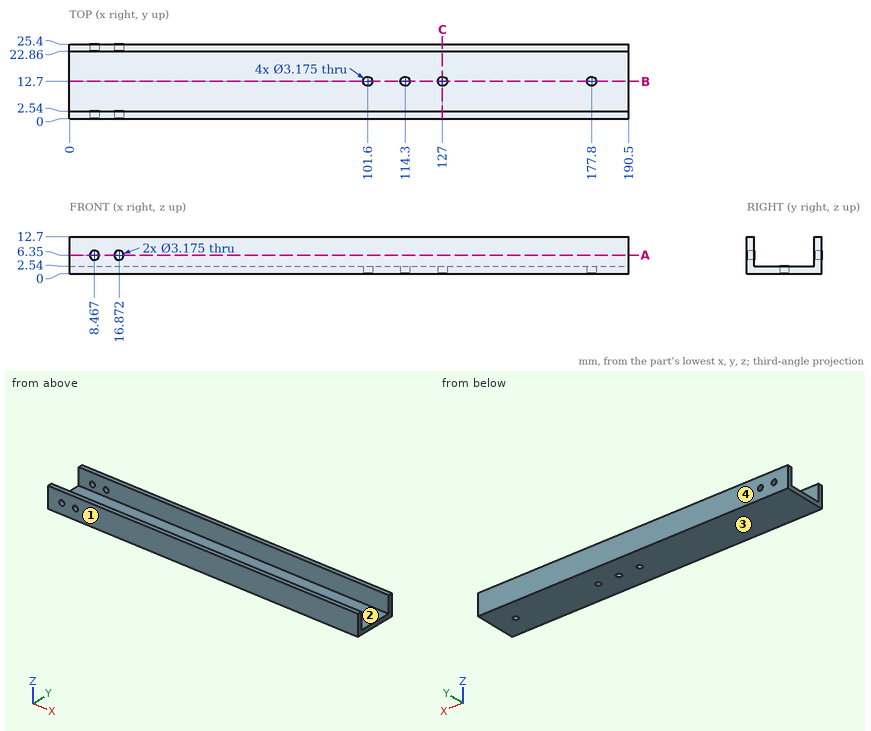
Geometry: see drawing. Coordinates: mm, zero at the bounding-box minimum. Give positions to 0.01 mm unless a question says otherwise; leave off trailing zeros. Order: outer loops, then holes, each group sorted by start corner. A loop starts at its lowest first (then second) coordinate and runs counter-clockwise, first axis right, second up. Notation, with made-up numbers: (50.5, 84) -> (54.5, 84) arc R23 ccw to (54.5, 122) -> close; hole circle Ø5 at (-4.5, -37.5). An arc over 180 degrees is marked (long way). Write each question's results on one line, items separated by ' | '. Start each with the question number.
1) Section A-A (z = 6.35). Return loops of the section in (x, y) (1 decimal).
2) Draft query along Y for the marked faces 1, 2, 3 and 4. Return one class per face: pulls with the +Y half, pulls with the -Y half, needs draft (parallel to the pull), parting line crosses it, or undercut.
3) Section C-C (x = 127). Return loops of the section in (y, z), then the cut area to 3 significant figures.
4) First-contact query: pin 1 (2.5 mm diameter, centred on x = 8.47, z = 6.35, fed in from +Y); pin 2 (6 mm diameter, centred on x = 110.5, y = 16, fed in from +Z). Flat tips, straight axial feed; report the tip coordinate or a pass-through.
5) Line query: line 1 (Y direction, x = 166, z = 12); line 2 (Y direction, x = 177.8, z = 1.9); line 3 (Z direction, x = 156, y = 12.5). Output: solid intervals per line, ascending. Write a range as from..to.
6) Section B-B (y = 12.7). Return loops of the section in (x, z).
Calculated:
1) outline: (0, 0) -> (6.9, 0) -> (6.9, 2.5) -> (0, 2.5) -> close; (0, 22.9) -> (6.9, 22.9) -> (6.9, 25.4) -> (0, 25.4) -> close; (10.1, 0) -> (15.3, 0) -> (15.3, 2.5) -> (10.1, 2.5) -> close; (10.1, 22.9) -> (15.3, 22.9) -> (15.3, 25.4) -> (10.1, 25.4) -> close; (18.5, 0) -> (190.5, 0) -> (190.5, 2.5) -> (18.5, 2.5) -> close; (18.5, 22.9) -> (190.5, 22.9) -> (190.5, 25.4) -> (18.5, 25.4) -> close
2) face 1: pulls with the -Y half | face 2: undercut | face 3: needs draft | face 4: pulls with the +Y half
3) outline: (0, 0) -> (11.11, 0) -> (11.11, 2.54) -> (2.54, 2.54) -> (2.54, 12.7) -> (0, 12.7) -> close; (14.29, 0) -> (25.4, 0) -> (25.4, 12.7) -> (22.86, 12.7) -> (22.86, 2.54) -> (14.29, 2.54) -> close | area: 108 mm2
4) pin 1: through | pin 2: z = 2.54
5) line 1: 0..2.54, 22.86..25.4 | line 2: 0..11.11, 14.29..25.4 | line 3: 0..2.54
6) outline: (0, 0) -> (100.01, 0) -> (100.01, 2.54) -> (0, 2.54) -> close; (103.19, 0) -> (112.71, 0) -> (112.71, 2.54) -> (103.19, 2.54) -> close; (115.89, 0) -> (125.41, 0) -> (125.41, 2.54) -> (115.89, 2.54) -> close; (128.59, 0) -> (176.21, 0) -> (176.21, 2.54) -> (128.59, 2.54) -> close; (179.39, 0) -> (190.5, 0) -> (190.5, 2.54) -> (179.39, 2.54) -> close
